from build123d import *

# Parameters (mm, degrees)
SKETCH2_R           = 6
BOSS_EXTRUDE1_DEPTH = 8
SKETCH3_R           = 27.5
SKETCH3_R_2         = 1.375
BOSS_EXTRUDE2_DEPTH = 10.5
SKETCH4_R           = 3
CUT_EXTRUDE1_DEPTH  = 9.5
CUT_EXTRUDE2_REACH  = 12.5


with BuildPart() as part:
    # Sketch2 → Boss-Extrude1 (new body)
    with BuildSketch(Plane(origin=(0, 0, 0), x_dir=(1, 0, 0), z_dir=(0, 1, 0))):
        Circle(SKETCH2_R)
        with BuildLine():
            ThreePointArc((-2, -1.887458609), (0, -2.75), (2, -1.887458609))
            Line((2, -1.887458609), (2, 1.887458609))
            ThreePointArc((2, 1.887458609), (0, 2.75), (-2, 1.887458609))
            Line((-2, 1.887458609), (-2, -1.887458609))
        make_face(mode=Mode.SUBTRACT)
    extrude(amount=BOSS_EXTRUDE1_DEPTH)

    # Sketch3 → Boss-Extrude2 (add)
    with BuildSketch(Plane(origin=(0, 0, 0), x_dir=(1, 0, 0), z_dir=(0, 1, 0))):
        Circle(SKETCH3_R)
        Circle(SKETCH3_R_2, mode=Mode.SUBTRACT)
        with BuildLine():
            Line((0, 6), (9.5, 22.454482672))
            ThreePointArc((9.5, 22.454482672), (0, 25), (-9.5, 22.454482672))
            Line((-9.5, 22.454482672), (0, 6))
        make_face(mode=Mode.SUBTRACT)
        with BuildLine():
            Line((4.690988895, 3.740938811), (11.632468358, 21.427540035))
            ThreePointArc((11.632468358, 21.427540035), (19.545787062, 15.587245046), (23.478774593, 6.572741869))
            Line((23.478774593, 6.572741869), (4.690988895, 3.740938811))
        make_face(mode=Mode.SUBTRACT)
        with BuildLine():
            Line((5.849567473, -1.335125604), (24.005450783, 4.26522271))
            ThreePointArc((24.005450783, 4.26522271), (24.373197805, -5.563023349), (19.777553038, -14.258407621))
            Line((19.777553038, -14.258407621), (5.849567473, -1.335125604))
        make_face(mode=Mode.SUBTRACT)
        with BuildLine():
            Line((2.603302435, -5.405813207), (18.301839147, -16.108894311))
            ThreePointArc((18.301839147, -16.108894311), (10.847093478, -22.524221698), (1.183430657, -24.352685354))
            Line((1.183430657, -24.352685354), (2.603302435, -5.405813207))
        make_face(mode=Mode.SUBTRACT)
        with BuildLine():
            Line((-2.603302435, -5.405813207), (-1.183430657, -24.352685354))
            ThreePointArc((-1.183430657, -24.352685354), (-10.847093478, -22.524221698), (-18.301839147, -16.108894311))
            Line((-18.301839147, -16.108894311), (-2.603302435, -5.405813207))
        make_face(mode=Mode.SUBTRACT)
        with BuildLine():
            Line((-5.849567473, -1.335125604), (-19.777553038, -14.258407621))
            ThreePointArc((-19.777553038, -14.258407621), (-24.373197805, -5.563023349), (-24.005450783, 4.26522271))
            Line((-24.005450783, 4.26522271), (-5.849567473, -1.335125604))
        make_face(mode=Mode.SUBTRACT)
        with BuildLine():
            Line((-4.690988895, 3.740938811), (-23.478774593, 6.572741868))
            ThreePointArc((-23.478774593, 6.572741868), (-19.545787062, 15.587245046), (-11.632468358, 21.427540035))
            Line((-11.632468358, 21.427540035), (-4.690988895, 3.740938811))
        make_face(mode=Mode.SUBTRACT)
    extrude(amount=-BOSS_EXTRUDE2_DEPTH)

    # Sketch4 → Cut-Extrude1 (cut)
    with BuildSketch(Plane(origin=(0, -10.5, 0), x_dir=(-1, 0, 0), z_dir=(0, -1, 0))):
        Circle(SKETCH4_R)
    extrude(amount=-CUT_EXTRUDE1_DEPTH, mode=Mode.SUBTRACT)

    # Sketch5 → Cut-Extrude2 (cut, up to next)
    with BuildSketch(Plane(origin=(0, 0, 0), x_dir=(1, 0, 0), z_dir=(0, 1, 0)), mode=Mode.PRIVATE) as cut_extrude2_sk1:
        with BuildLine():
            ThreePointArc((-5.206364569, -4.698553628), (-5.138695362, -4.097972805), (-5.739276185, -4.030303598))
            Line((-5.739276185, -4.030303598), (-16.68491694, -12.759160824))
            ThreePointArc((-16.68491694, -12.759160824), (-16.752586147, -13.359741647), (-16.152005324, -13.427410854))
            Line((-16.152005324, -13.427410854), (-5.206364569, -4.698553628))
        make_face()
    cut_extrude2_tool1 = extrude(cut_extrude2_sk1.sketch, amount=-CUT_EXTRUDE2_REACH, mode=Mode.PRIVATE) & part.part
    add(cut_extrude2_tool1.solids().sort_by_distance((-10.945641, 0, 8.728857))[0], mode=Mode.SUBTRACT)
    # Sketch5 → Cut-Extrude2 (cut, up to next)
    with BuildSketch(Plane(origin=(0, 0, 0), x_dir=(1, 0, 0), z_dir=(0, 1, 0)), mode=Mode.PRIVATE) as cut_extrude2_sk2:
        with BuildLine():
            Line((0.427361935, -21), (0.427361935, -7))
            ThreePointArc((0.427361935, -7), (0, -6.572638065), (-0.427361935, -7))
            Line((-0.427361935, -7), (-0.427361935, -21))
            ThreePointArc((-0.427361935, -21), (0, -21.427361935), (0.427361935, -21))
        make_face()
    cut_extrude2_tool2 = extrude(cut_extrude2_sk2.sketch, amount=-CUT_EXTRUDE2_REACH, mode=Mode.PRIVATE) & part.part
    add(cut_extrude2_tool2.solids().sort_by_distance((0, 0, 14))[0], mode=Mode.SUBTRACT)
    # Sketch5 → Cut-Extrude2 (cut, up to next)
    with BuildSketch(Plane(origin=(0, 0, 0), x_dir=(1, 0, 0), z_dir=(0, 1, 0)), mode=Mode.PRIVATE) as cut_extrude2_sk3:
        with BuildLine():
            ThreePointArc((-6.919592362, 1.140999459), (-6.407848306, 1.462549561), (-6.729398408, 1.974293617))
            Line((-6.729398408, 1.974293617), (-20.378389179, 5.089586692))
            ThreePointArc((-20.378389179, 5.089586692), (-20.890133235, 4.76803659), (-20.568583133, 4.256292534))
            Line((-20.568583133, 4.256292534), (-6.919592362, 1.140999459))
        make_face()
    cut_extrude2_tool3 = extrude(cut_extrude2_sk3.sketch, amount=-CUT_EXTRUDE2_REACH, mode=Mode.PRIVATE) & part.part
    add(cut_extrude2_tool3.solids().sort_by_distance((-13.648991, 0, -3.115293))[0], mode=Mode.SUBTRACT)
    # Sketch5 → Cut-Extrude2 (cut, up to next)
    with BuildSketch(Plane(origin=(0, 0, 0), x_dir=(1, 0, 0), z_dir=(0, 1, 0)), mode=Mode.PRIVATE) as cut_extrude2_sk4:
        with BuildLine():
            ThreePointArc((-3.422225972, 6.121356681), (-2.85176078, 5.921742277), (-2.652146375, 6.49220747))
            Line((-2.652146375, 6.49220747), (-8.726518723, 19.10577162))
            ThreePointArc((-8.726518723, 19.10577162), (-9.296983916, 19.305386025), (-9.49659832, 18.734920832))
            Line((-9.49659832, 18.734920832), (-3.422225972, 6.121356681))
        make_face()
    cut_extrude2_tool4 = extrude(cut_extrude2_sk4.sketch, amount=-CUT_EXTRUDE2_REACH, mode=Mode.PRIVATE) & part.part
    add(cut_extrude2_tool4.solids().sort_by_distance((-6.074372, 0, -12.613564))[0], mode=Mode.SUBTRACT)
    # Sketch5 → Cut-Extrude2 (cut, up to next)
    with BuildSketch(Plane(origin=(0, 0, 0), x_dir=(1, 0, 0), z_dir=(0, 1, 0)), mode=Mode.PRIVATE) as cut_extrude2_sk5:
        with BuildLine():
            ThreePointArc((2.652146375, 6.49220747), (2.85176078, 5.921742277), (3.422225972, 6.121356681))
            Line((3.422225972, 6.121356681), (9.49659832, 18.734920832))
            ThreePointArc((9.49659832, 18.734920832), (9.296983916, 19.305386025), (8.726518723, 19.10577162))
            Line((8.726518723, 19.10577162), (2.652146375, 6.49220747))
        make_face()
    cut_extrude2_tool5 = extrude(cut_extrude2_sk5.sketch, amount=-CUT_EXTRUDE2_REACH, mode=Mode.PRIVATE) & part.part
    add(cut_extrude2_tool5.solids().sort_by_distance((6.074372, 0, -12.613564))[0], mode=Mode.SUBTRACT)
    # Sketch5 → Cut-Extrude2 (cut, up to next)
    with BuildSketch(Plane(origin=(0, 0, 0), x_dir=(1, 0, 0), z_dir=(0, 1, 0)), mode=Mode.PRIVATE) as cut_extrude2_sk6:
        with BuildLine():
            ThreePointArc((6.729398408, 1.974293617), (6.407848306, 1.462549561), (6.919592362, 1.140999459))
            Line((6.919592362, 1.140999459), (20.568583133, 4.256292534))
            ThreePointArc((20.568583133, 4.256292534), (20.890133235, 4.76803659), (20.378389179, 5.089586692))
            Line((20.378389179, 5.089586692), (6.729398408, 1.974293617))
        make_face()
    cut_extrude2_tool6 = extrude(cut_extrude2_sk6.sketch, amount=-CUT_EXTRUDE2_REACH, mode=Mode.PRIVATE) & part.part
    add(cut_extrude2_tool6.solids().sort_by_distance((13.648991, 0, -3.115293))[0], mode=Mode.SUBTRACT)
    # Sketch5 → Cut-Extrude2 (cut, up to next)
    with BuildSketch(Plane(origin=(0, 0, 0), x_dir=(1, 0, 0), z_dir=(0, 1, 0)), mode=Mode.PRIVATE) as cut_extrude2_sk7:
        with BuildLine():
            ThreePointArc((5.739276185, -4.030303598), (5.138695362, -4.097972805), (5.206364569, -4.698553628))
            Line((5.206364569, -4.698553628), (16.152005324, -13.427410854))
            ThreePointArc((16.152005324, -13.427410854), (16.752586147, -13.359741647), (16.68491694, -12.759160824))
            Line((16.68491694, -12.759160824), (5.739276185, -4.030303598))
        make_face()
    cut_extrude2_tool7 = extrude(cut_extrude2_sk7.sketch, amount=-CUT_EXTRUDE2_REACH, mode=Mode.PRIVATE) & part.part
    add(cut_extrude2_tool7.solids().sort_by_distance((10.945641, 0, 8.728857))[0], mode=Mode.SUBTRACT)


solid = part.part
CAD build for the part. Positions are in the model's coordinates, mm. A direction names the side the tool comes from. Round coordinates to 2 decimals unless told otherwise and drop trailing zeros. Write each loop counter-clockwise with the first axis right and the second up, starting at its lowest first coordinate (ties: lowest second). Pieces come first, ordered by that corner, then holes. Notation, with made-up numbers: M -13,54 L 23,54 A34 ccw 23,91 Z; hole C 71,17.5 d3. An arc over 180 degrees is marked long. Use a Markdown table: item, result. Add a question column.
1. Flat gauge pins, fed straight in: P1, Ø10, axis at x = 17, y = -4, coming from the +Z side; P2, Ø6, axis at y = 3.5, z = -7.5, coming from the +X side; P3, Ø8, axis at x = -12.5, y = -3.5, coming from the +Z side. Where does each tip first touch, or does it go through?
2. Slice it at A-A on z = 0. Give the cut face in (x, y) (3 decimals).
3. 3-axis set-ups, long thin cutter, end or side, ignore diameter. For faces 1 (the face through (1.883, -5.176, 15.012)), 2 (the face through (2, 4, 0)): which of +Z, -Z, +X, -X, +Y, -Y reach the whole face in a straight line?
4. Drill centre lines: probe 1 along Z at (x, y) = (-19, -8); probe 2 along X at (y, z) = (-2.5, 5); probe 3 along Y at (x, z) = (-25, 0). Where is each one in solid material? Low to high.
5. Slice it at B-B on y = 5.5. Give the cut face in (x, z), then the cut area to 3 significant figures.
6. Slice it at C-C on z = -9. Give the cut face in (x, y).
7. Slice it at D-D on y = -4.25. Give the number of separate pieces and of enclosed holes in the cut face, then the cut area to 3 significant figures.
Reply:
| question | item | result |
|---|---|---|
| 1 | P1 | stops at z = 24.74 |
| 1 | P2 | stops at x = 3.97 |
| 1 | P3 | stops at z = 26.15 |
| 2 | outline | M -27.5,-10.5 L -24.803,-10.5 L -24.803,0 L -27.5,0 Z; M -10.178,-10.5 L -3,-10.5 L -3,-1 L -1.375,-1 L -1.375,0 L -2,0 L -2,8 L -6,8 L -6,0 L -10.178,0 Z; M 1.375,-1 L 3,-1 L 3,-10.5 L 10.178,-10.5 L 10.178,0 L 6,0 L 6,8 L 2,8 L 2,0 L 1.375,0 Z; M 24.803,-10.5 L 27.5,-10.5 L 27.5,0 L 24.803,0 Z |
| 3 | face 1 | +Y, -Y |
| 3 | face 2 | +Y |
| 4 | probe 1 | z = -19.88 to -16.24, -5.9 to -4.77, -3.9 to -2.72, 13.54 to 19.88 |
| 4 | probe 2 | x = -27.04 to -24.49, -9.8 to -6.96, -5.58 to 5.58, 6.96 to 9.8, 24.49 to 27.04 |
| 4 | probe 3 | y = -10.5 to 0 |
| 5 | outline | C 0,0 d12; hole M -2,-1.89 A2.75 ccw 2,-1.89 L 2,1.89 A2.75 ccw -2,1.89 Z |
| 5 | area | 93.2 mm^2 |
| 6 | outline | M -25.99,-10.5 L -22.95,-10.5 L -22.95,0 L -25.99,0 Z; M -6.76,-10.5 L -4.81,-10.5 L -4.81,0 L -6.76,0 Z; M -3.86,-10.5 L -1.73,-10.5 L -1.73,0 L -3.86,0 Z; M 1.73,-10.5 L 3.86,-10.5 L 3.86,0 L 1.73,0 Z; M 4.81,-10.5 L 6.76,-10.5 L 6.76,0 L 4.81,0 Z; M 22.95,-10.5 L 25.99,-10.5 L 25.99,0 L 22.95,0 Z |
| 7 | separate pieces | 1 |
| 7 | enclosed holes | 15 |
| 7 | area | 937 mm^2 |
